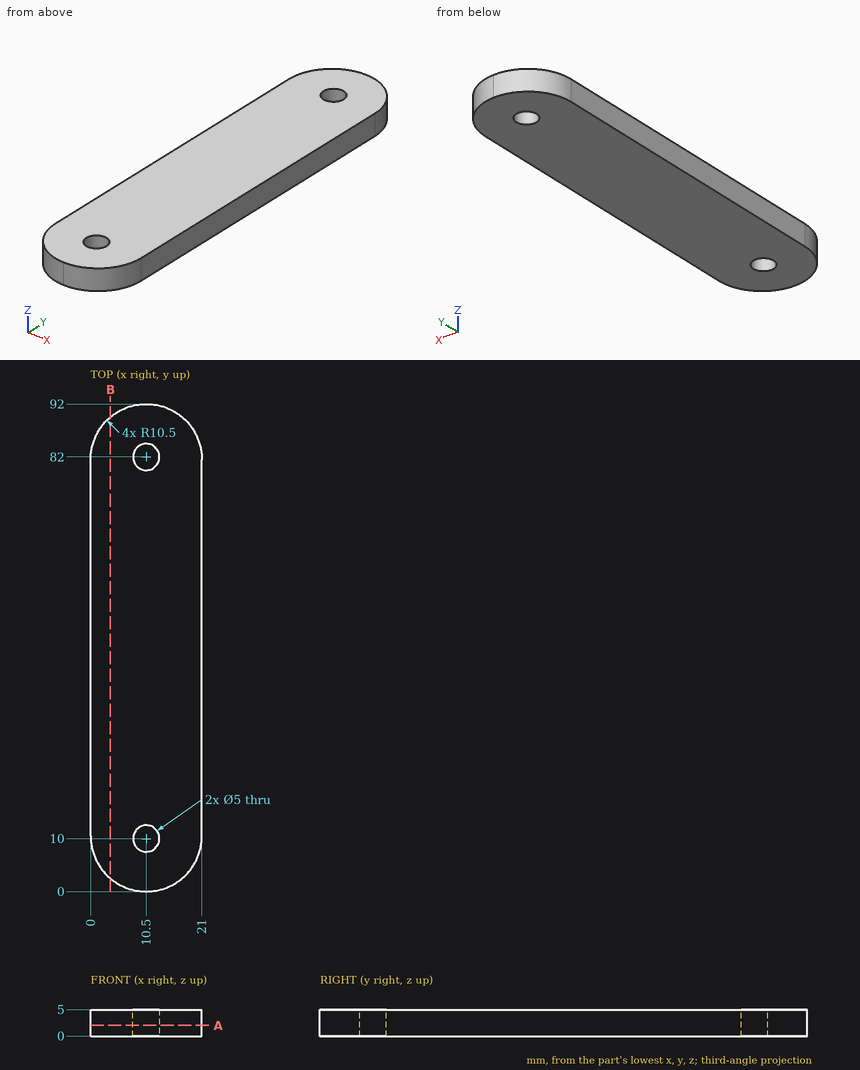
Job drawing, mm, ordinate dimensions from the low corner. One solid piece. Give positions to 0.01 mm unless a question says otherwise; leave off trailing zeros. Loops run counter-clockwise (first coordinate to the right, second up) from the corner with the lowest first, then second, coordinate; pieces in that order, holes last. Notation, with made-up numbers: (24.5, 41) -> (74.5, 41) arc R24 cw to (74.5, 68) -> close; hole circle Ø5 at (-32.5, -5). An arc over 180 degrees is marked (long way). Use a Markdown table: item, result. Add a question column.
(1) Slice it at B-B on x = 3.75. List the corners of the cut face in (y, z).
(2) Wall check: line 1 along Y through (x, z) = (10.5, 2.25); line 2 along Y through (x, z) = (8.5, 0.9); line 3 along X through (y, z) = (80, 4.8). Give the ranges that are in metal, low to high.
(3) Slice it at A-A on z = 2. Give the number of separate pieces and of enclosed holes in the cut face, and give its area (3 significant figures).
(4) Drop a flat-ended pin along its axis: pin 1 Ø1 at (x, z) = (8, 4) entering from +Y. Give the stop position or say it passes through.
Filled sheet:
| question | item | result |
|---|---|---|
| 1 | outline | (2.46, 0) -> (89.54, 0) -> (89.54, 5) -> (2.46, 5) -> close |
| 2 | line 1 | 0 to 7.5, 12.5 to 79.5, 84.5 to 92 |
| 2 | line 2 | 0.19 to 8.5, 11.5 to 80.5, 83.5 to 91.81 |
| 2 | line 3 | 0 to 9, 12 to 21 |
| 3 | separate pieces | 1 |
| 3 | enclosed holes | 2 |
| 3 | area | 1,800 mm2 |
| 4 | pin 1 | y = 91.81 |
